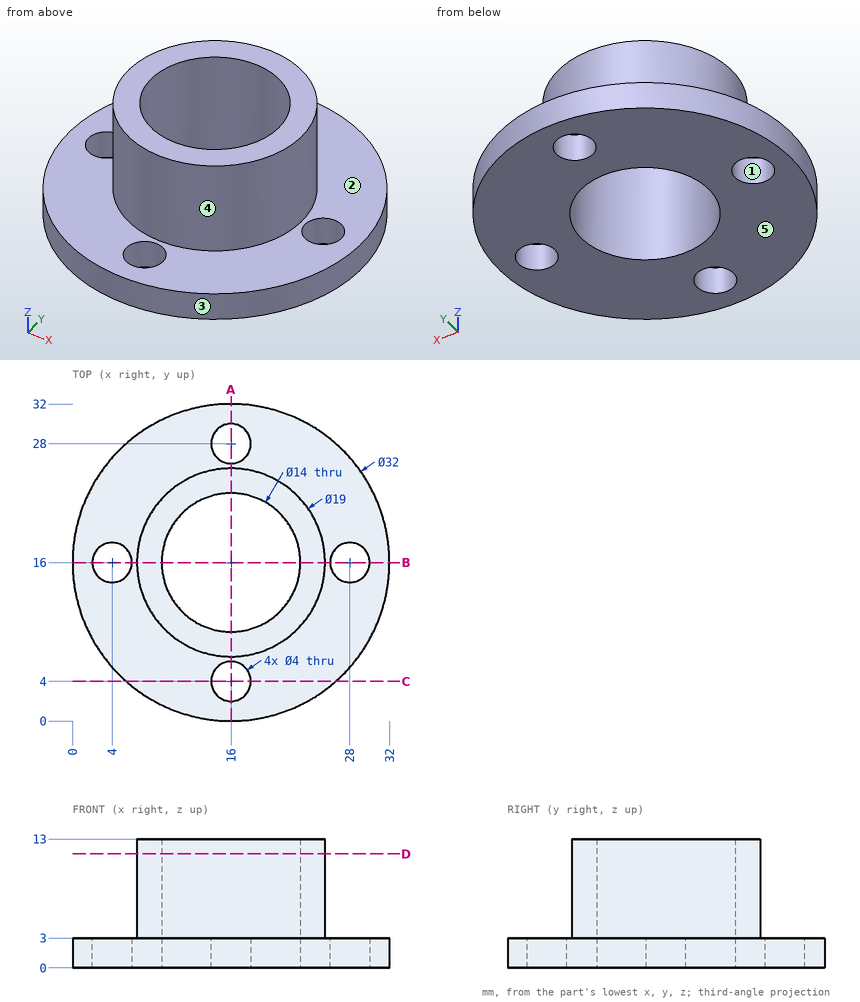
Geometry: see drawing. Coordinates: mm, zero at the bounding-box minimum. A direction names the side the tool comes from. Round coordinates to 2 decimals unless told otherwise and drop trailing zeros. Loops run counter-clockwise (first coordinate to the right, second up) from the corner with the lowest first, then second, coordinate; pieces in that order, holes last. Notation, with made-up numbers: (36, -34.75) -> (56, -34.75) arc R22 cw to (56, 0.25) -> close; hole circle Ø11 at (13.5, 19). An arc over 180 degrees is marked (long way). Use one line per item in the form item = value. Start each with the question number.
Item 1: Material intervals for L1, parallel to Y at x = 16, z = 1.25; L2, parallel to Y at x = 16, z = 7.25; L3, parallel to Z at x = 5.5, y = 11, sorted ascending. Write a range as from..to.
Item 2: Section query D-D on z = 11.5. Return the cut outline in (x, y), then the cut area to 3 significant figures.
Item 3: Section query A-A on x = 16. Return the cut outline in (y, z).
Item 4: Mould query, pull axis X, two halves, no side actions, for the marked faces 1, 2 and 3. Classes: pulls with the +X half, pulls with the -X half, needs draft (parallel to the pull), parting line crosses it, or undercut.
Item 5: Set-up query: the marked faces 4 and 5. Return all of +Z, -Z, +X, -X, +Y, -Y with unobstructed straight access to the full face (end or side cutting, diameter ignored); none if empty.
Item 6: Contact query for a flat-ended pin moving along its axis: pin 1 Ø4.5 at (x, y) = (28, 16) entering from +Z. Output: stop coordinate, or through.
Item 7: Section query C-C on y = 4. Return the cut outline in (x, z), then the cut area to 3 significant figures.
Ans:
q1.L1 = 0..2, 6..9, 23..26, 30..32
q1.L2 = 6.5..9, 23..25.5
q1.L3 = 0..3
q2.outline = circle Ø19 at (16, 16); hole circle Ø14 at (16, 16)
q2.area = 130 mm^2
q3.outline = (0, 0) -> (2, 0) -> (2, 3) -> (0, 3) -> close; (6, 0) -> (9, 0) -> (9, 13) -> (6.5, 13) -> (6.5, 3) -> (6, 3) -> close; (23, 0) -> (26, 0) -> (26, 3) -> (25.5, 3) -> (25.5, 13) -> (23, 13) -> close; (30, 0) -> (32, 0) -> (32, 3) -> (30, 3) -> close
q4.face_1 = undercut
q4.face_2 = needs draft
q4.face_3 = parting line crosses it
q5.face_4 = +Z
q5.face_5 = -Z, +X, -X, +Y, -Y
q6.pin_1 = 3
q7.outline = (5.42, 0) -> (14, 0) -> (14, 3) -> (5.42, 3) -> close; (18, 0) -> (26.58, 0) -> (26.58, 3) -> (18, 3) -> close
q7.area = 51.5 mm^2
